```python
from build123d import *

# Parameters (mm, degrees)
SKETCH1_W        = 26
SKETCH1_H        = 31
SKETCH1_R        = 4.8
SKETCH1_R_2      = 2
SKETCH1_R_3      = 1
EXTRUSION1_DEPTH = 2
SKETCH2_W        = 26
SKETCH2_H        = 2
EXTRUSION2_DEPTH = 34
SKETCH3_R        = 1.6
SKETCH3_R_2      = 4
SKETCH3_R_3      = 0.0001
EXTRUSION3_DEPTH = 34
FILLET1_R        = 2
FILLET2_R        = 2


with BuildPart() as part:
    # Sketch1 → Extrusion1 (new body)
    with BuildSketch(Plane(origin=(0, 0, 0), x_dir=(-1, 0, 0), z_dir=(0, 1, 0))):
        Rectangle(SKETCH1_W, SKETCH1_H)
        with Locations(Location((0, 0, 0), (0, 0, 90))):
            Circle(SKETCH1_R, mode=Mode.SUBTRACT)
        with Locations(Location((7, 8, 0), (0, 0, 90))):
            Circle(SKETCH1_R_2, mode=Mode.SUBTRACT)
        with Locations(Location((7, -8, 0), (0, 0, 90))):
            Circle(SKETCH1_R_2, mode=Mode.SUBTRACT)
        with Locations(Location((-7, -8, 0), (0, 0, 90))):
            Circle(SKETCH1_R_2, mode=Mode.SUBTRACT)
        with Locations(Location((-7, 8, 0), (0, 0, 90))):
            Circle(SKETCH1_R_2, mode=Mode.SUBTRACT)
        with Locations(Location((0, 10, 0), (0, 0, 90))):
            Circle(SKETCH1_R_3, mode=Mode.SUBTRACT)
        with Locations(Location((0, -10, 0), (0, 0, 90))):
            Circle(SKETCH1_R_3, mode=Mode.SUBTRACT)
    extrude(amount=EXTRUSION1_DEPTH)

    # Sketch2 → Extrusion2 (add)
    with BuildSketch(Plane(origin=(0, 0, 0), x_dir=(-1, 0, 0), z_dir=(0, 1, 0))):
        with Locations((0, -16.5)):
            Rectangle(SKETCH2_W, SKETCH2_H)
    extrude(amount=EXTRUSION2_DEPTH)

    # Sketch3 → Extrusion3 (cut)
    with BuildSketch(Plane.XY.offset(-15.5)):
        with Locations((0, 29.5)):
            Circle(SKETCH3_R)
        with Locations((8.5, 21)):
            Circle(SKETCH3_R)
        with Locations((0, 12.5)):
            Circle(SKETCH3_R)
        with Locations((-8.5, 21)):
            Circle(SKETCH3_R)
        with Locations((0, 21)):
            Circle(SKETCH3_R_2)
        with Locations((-0.072111026, 33.9999)):
            Circle(SKETCH3_R_3)
        with Locations((0.072111026, 33.9999)):
            Circle(SKETCH3_R_3)
        with BuildLine():
            Line((-0.072111026, 34), (-13, 34))
            Line((-13, 34), (-13, 21))
            ThreePointArc((-13, 21), (-9.2178478, 30.166857801), (-0.072111026, 34))
        make_face()
        with BuildLine():
            Line((13, 21), (13, 34))
            Line((13, 34), (0.072111026, 34))
            ThreePointArc((0.072111026, 34), (9.2178478, 30.166857801), (13, 21))
        make_face()
    extrude(amount=-EXTRUSION3_DEPTH, mode=Mode.SUBTRACT)

    # Fillet1
    fillet1_edges = [part.edges().sort_by_distance(p)[0] for p in [
        (0, 0, -17.5),
    ]]
    fillet(fillet1_edges, radius=FILLET1_R)

    # Fillet2
    fillet2_edges = [part.edges().sort_by_distance(p)[0] for p in [
        (-13, 1, 15.5),
        (13, 1, 15.5),
    ]]
    fillet(fillet2_edges, radius=FILLET2_R)


solid = part.part
```
For this review, take the finished solid that the model builds, in its own axes (mm). A direction names the side the tool comes from. Round coordinates to 2 decimals unless told otherwise and drop trailing zeros. Write each loop counter-clockwise with the first axis right and the second up, starting at its lowest first coordinate (ties: lowest second). Pieces come first, ordered by that corner, then holes. Notation, with made-up numbers: (-24.75, -18) -> (-13.75, -18) arc R20 cw to (-13.75, 19) -> close; hole circle Ø4 at (55.25, 16). An arc over 180 degrees is marked (long way). Use one line per item in the form item = value.
1) Take a section at A-A, the plane z = -8. Write out the cut boundary in (x, y), and give its area (3 significant figures).
Found:
outline = (-13, 0) -> (-9, 0) -> (-9, 2) -> (-13, 2) -> close; (-5, 0) -> (5, 0) -> (5, 2) -> (-5, 2) -> close; (9, 0) -> (13, 0) -> (13, 2) -> (9, 2) -> close
area = 36.0 mm2
2) Take a section at B-B, the plane z = 0. Write out the cut boundary in (x, y), and give its area (3 significant figures).
Found:
outline = (-13, 0) -> (-4.8, 0) -> (-4.8, 2) -> (-13, 2) -> close; (4.8, 0) -> (13, 0) -> (13, 2) -> (4.8, 2) -> close
area = 32.8 mm2
3) Mouldability with a two-part tool opening along X and no side actions: class faces 3 (the cylindrical face through (-12.4, 1.01, 14.93)), 4 (the flat face through (0, 1, 15.5)), 5 (the cylindrical face through (-0.6, 1, -10.8)) as +X half, -X half, draft (parallel to the pull), parting line (faces both ways), or undercut.
Found:
face_3 = -X half
face_4 = draft
face_5 = undercut
4) Clearance check with flat-ended pins moving along their axes: pin 1 (10 mm diameter, centred on x = -3, y = 30, fed in from +Z); pin 2 (1.8 mm diameter, centred on x = 0, z = -10, fed in from +Y); pin 3 (8 mm diameter, centred on x = 5, z = 0, fed in from +Y). State where each tip first meets the part, or that it passes through.
Found:
pin_1 = -15.5
pin_2 = through
pin_3 = 2
5) Take a section at C-C, the plane y = 12.5. Write out the cut boundary in (x, z), and give its area (3 significant figures).
Found:
outline = (-13, -17.5) -> (-1.6, -17.5) -> (-1.6, -15.5) -> (-13, -15.5) -> close; (1.6, -17.5) -> (13, -17.5) -> (13, -15.5) -> (1.6, -15.5) -> close
area = 45.6 mm2
6) To check wall thickness, follow L1, parallel to X at y = 1.2, z = 8; L2, parallel to Y at x = 0, z = -16.9; L3, parallel to Z at x = -11, y = 13.5. State the ranges of each line that lie inside material, in increasing order. Write a range as from..to.
Found:
L1 = -13..-9, -5..5, 9..13
L2 = 0.57..10.9, 14.1..17, 25..27.9, 31.1..34
L3 = -17.5..-15.5
7) Take a section at D-D, the plane x = -8.25. Write out the cut boundary in (y, z).
Found:
outline = (0, -15.5) arc R2 ccw to (2, -17.5) -> (19.42, -17.5) -> (19.42, -15.5) -> (2, -15.5) -> (2, -9.56) -> (0, -9.56) -> close; (0, -6.44) -> (2, -6.44) -> (2, 6.44) -> (0, 6.44) -> close; (0, 9.56) -> (2, 9.56) -> (2, 15.5) -> (0, 15.5) -> close; (22.58, -17.5) -> (31.05, -17.5) -> (31.05, -15.5) -> (22.58, -15.5) -> close
8) Tool access review of faces 1 (the flat face through (-3, 18, -15.5)), 2 (the cylindrical face through (9.117, 30.267, -16.486)): name each direction out of +Z, -Z, +X, -X, +Y, -Y from which nothing blocks a thin tool from reaching the whole face with its end or side.
Found:
face_1 = +Z, +X, -X, +Y
face_2 = +Z, -Z, +X, +Y
